from build123d import *

# Parameters (mm, degrees)
SKETCH_1_R      = 3.55
EXTRUDE_1_DEPTH = 3


with BuildPart() as part:
    # 草图1 → 凸台-拉伸1 (new body)
    with BuildSketch(Plane.XY.offset(3)):
        Polygon((46.131858504, 44.9999), (19.632388504, 44.9999), (19.632388504, 35.9998), (16.632358504, 35.9998), (16.632358504, 44.9999), (-3.867371496, 44.9999), (-3.867371496, 29.9998), (-0.867341496, 29.9998), (-0.867341496, 9.9991), (-3.867371496, 9.9991), (-3.867371496, 0), (16.632358504, 0), (16.632358504, 7.4993), (19.632388504, 7.4993), (19.632388504, 0), (46.131858504, 0), (46.131858504, 13.0005), (43.131858504, 13.0005), (43.131858504, 34.9994), (46.131858504, 34.9994), align=None)
        with Locations(Location((21.131658504, 22.4992, 0), (0, 0, 180))):
            Circle(SKETCH_1_R, mode=Mode.SUBTRACT)
        with BuildLine():
            Line((9.236684618, 23.399), (14.226589495, 23.399))
            ThreePointArc((14.226589495, 23.399), (15.126339495, 22.49925), (14.226589495, 21.5995))
            Line((14.226589495, 21.5995), (9.236684618, 21.5995))
            ThreePointArc((9.236684618, 21.5995), (8.336934618, 22.49925), (9.236684618, 23.399))
        make_face(mode=Mode.SUBTRACT)
        with BuildLine():
            Line((33.064389495, 21.5871), (28.074484618, 21.5871))
            ThreePointArc((28.074484618, 21.5871), (27.174734618, 22.48685), (28.074484618, 23.3866))
            Line((28.074484618, 23.3866), (33.064389495, 23.3866))
            ThreePointArc((33.064389495, 23.3866), (33.964139495, 22.48685), (33.064389495, 21.5871))
        make_face(mode=Mode.SUBTRACT)
    extrude(amount=-EXTRUDE_1_DEPTH)


solid = part.part
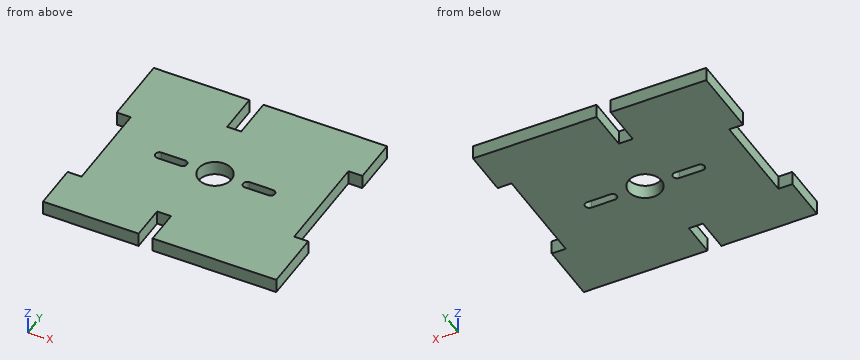
Build history of the part. All positions in model axes, mm. Give positions to 0.01 mm unless a question says otherwise; leave off trailing zeros. Loops run counter-clockwise (first coordinate to the right, second up) from the corner with the lowest first, then second, coordinate; pieces in that order, holes last. Notation, with made-up numbers: (44, 75.5) - (87, 75.5) arc R21 ccw to (87, 85.5) - close; hole circle Ø4 at (-35.5, 36.5). An arc over 180 degrees is marked (long way). Write item = value, one per line. Start each with the question number.
1) Drop flat-ended pins along their axis: pin 1 Ø8 at (x, y) = (21.13, 22.5) entering from +Z; pin 2 Ø1.5 at (y, z) = (22, 1.5) entering from -X; pin 3 Ø1.5 at (y, z) = (25.5, 1) entering from +X; pin 4 Ø1.5 at (x, z) = (18.5, 2) entering from -Y. Give the stop position or say it passes through.
2) Probe probe 1 along X at (y, z) = (43, 0.1); probe 2 along Y at (x, z) = (31.5, 1.45); probe 3 along Y at (x, z) = (21, 0.7). List the from-to ranges inside material, lowest first. Write a range as from..to.
3) Band-saw the part on A-A on y = 5.5. Give the cut face in (x, z), plus the area to 3 significant figures.
4) Band-saw the part on B-B on z = 2.05. Count the separate pieces of the cut face and the enclosed holes in it, plus the area to 3 significant figures.
Final values:
q1.pin_1 = 3
q1.pin_2 = -0.87
q1.pin_3 = 43.13
q1.pin_4 = 7.5
q2.probe_1 = -3.87..16.63, 19.63..46.13
q2.probe_2 = 0..21.59, 23.39..45
q2.probe_3 = 0..18.95, 26.05..45
q3.outline = (-3.87, 0) - (16.63, 0) - (16.63, 3) - (-3.87, 3) - close; (19.63, 0) - (46.13, 0) - (46.13, 3) - (19.63, 3) - close
q3.area = 141 mm²
q4.separate_pieces = 1
q4.enclosed_holes = 3
q4.area = 2,010 mm²
